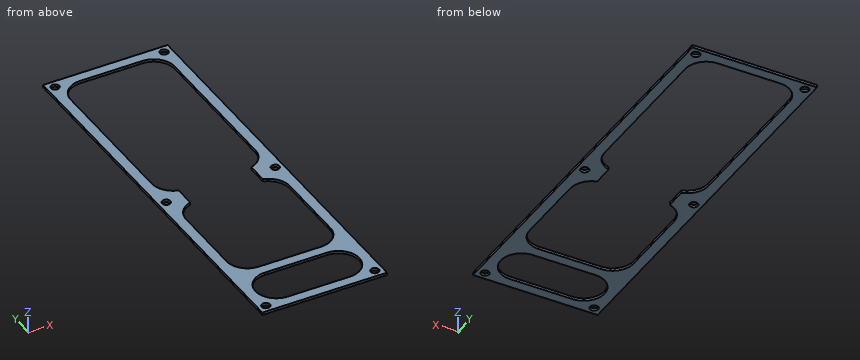
from build123d import *

# Parameters (mm, degrees)
SKETCH1_W           = 76.2
SKETCH1_H           = 241.3
BOSS_EXTRUDE1_DEPTH = 1.5875
CUT_EXTRUDE1_DEPTH  = 1.5875
SKETCH3_R           = 2.4892
CUT_EXTRUDE2_DEPTH  = 1.5875


with BuildPart() as part:
    # Sketch1 → Boss-Extrude1 (new body)
    with BuildSketch(Plane.XY):
        with Locations((38.1, -120.65)):
            Rectangle(SKETCH1_W, SKETCH1_H)
    extrude(amount=BOSS_EXTRUDE1_DEPTH)

    # Sketch2 → Cut-Extrude1 (cut)
    with BuildSketch(Plane.XY.offset(1.5875)):
        with BuildLine():
            Line((19.05, -6.35), (57.15, -6.35))
            ThreePointArc((57.15, -6.35), (66.130256121, -10.069743879), (69.85, -19.05))
            Line((69.85, -19.05), (69.85, -107.95))
            ThreePointArc((69.85, -107.95), (67.204166667, -115.8875), (60.325, -120.65))
            Line((60.325, -120.65), (60.325, -133.35))
            ThreePointArc((60.325, -133.35), (67.204166667, -138.1125), (69.85, -146.05))
            Line((69.85, -146.05), (69.85, -190.5))
            ThreePointArc((69.85, -190.5), (66.130256121, -199.480256121), (57.15, -203.2))
            Line((57.15, -203.2), (19.05, -203.2))
            ThreePointArc((19.05, -203.2), (10.069743879, -199.480256121), (6.35, -190.5))
            Line((6.35, -190.5), (6.35, -146.05))
            ThreePointArc((6.35, -146.05), (8.995833333, -138.1125), (15.875, -133.35))
            Line((15.875, -133.35), (15.875, -120.65))
            ThreePointArc((15.875, -120.65), (8.995833333, -115.8875), (6.35, -107.95))
            Line((6.35, -107.95), (6.35, -19.05))
            ThreePointArc((6.35, -19.05), (10.069743879, -10.069743879), (19.05, -6.35))
        make_face()
        with BuildLine():
            Line((19.05, -234.95), (57.15, -234.95))
            ThreePointArc((57.15, -234.95), (69.85, -222.25), (57.15, -209.55))
            Line((57.15, -209.55), (19.05, -209.55))
            ThreePointArc((19.05, -209.55), (6.35, -222.25), (19.05, -234.95))
        make_face()
    extrude(amount=-CUT_EXTRUDE1_DEPTH, mode=Mode.SUBTRACT)

    # Sketch3 → Cut-Extrude2 (cut)
    with BuildSketch(Plane.XY.offset(1.5875)):
        with Locations((4.7625, -4.7625)):
            Circle(SKETCH3_R)
        with Locations((71.4375, -4.7625)):
            Circle(SKETCH3_R)
        with Locations((71.4375, -127)):
            Circle(SKETCH3_R)
        with Locations((4.7625, -127)):
            Circle(SKETCH3_R)
        with Locations((4.7625, -236.5375)):
            Circle(SKETCH3_R)
        with Locations((71.4375, -236.5375)):
            Circle(SKETCH3_R)
    extrude(amount=-CUT_EXTRUDE2_DEPTH, mode=Mode.SUBTRACT)


solid = part.part
Input: part model. Units: mm. Frame: model coordinates. Coordinates: 2 decimals unless noted, no trailing zeros. Order: outer loops, then holes, each group sorted by start corner. A loop starts at its lowest first (then second) coordinate and runs counter-clockwise, first axis right, second up. Notation, with made-up numbers: M 31.5,10 L 40.5,10 A12 ccw 40.5,14 Z; hole C -25.75,74 d1. An arc over 180 degrees is marked long. One line per question, with ' | ' between items.
Item 1: Ray query, line 1 along Y through (x, z) = (44.5, 0.3); line 2 along Y through (x, z) = (5, 0.75); line 3 along X through (y, z) = (-26.5, 0.65). Return the intervals inside material, ascending.
Geometry results:
line 1: y = -241.3 to -234.95, -209.55 to -203.2, -6.35 to 0 | line 2: y = -241.3 to -239.02, -234.06 to -129.48, -124.52 to -7.24, -2.28 to 0 | line 3: x = 0 to 6.35, 69.85 to 76.2
Item 2: Section A-A (y = -222.25). Output: boundary loops of the cut face in (x, z).
Geometry results:
outline: M 0,0 L 6.35,0 L 6.35,1.59 L 0,1.59 Z; M 69.85,0 L 76.2,0 L 76.2,1.59 L 69.85,1.59 Z
Item 3: Section B-B (y = -127). Output: boundary loops of the cut face in (x, z) (1 decimal), then the cut area to 3 significant figures.
Geometry results:
outline: M 0,0 L 2.3,0 L 2.3,1.6 L 0,1.6 Z; M 7.3,0 L 15.9,0 L 15.9,1.6 L 7.3,1.6 Z; M 60.3,0 L 68.9,0 L 68.9,1.6 L 60.3,1.6 Z; M 73.9,0 L 76.2,0 L 76.2,1.6 L 73.9,1.6 Z | area: 34.6 mm^2
Item 4: Section C-C (z = 0.7). Give the number of separate pieces and of enclosed holes in the cut face, then the cut area to 3 significant figures.
Geometry results:
separate pieces: 1 | enclosed holes: 8 | area: 4,800 mm^2
Item 5: Pin query (flat end, axial travel): pin 1 (3 mm diameter, centred on x = 55, y = -212, fed in from -Z). Return the tip coordinate at first contact, or that it passes through.
Geometry results:
pin 1: passes through
